```python
from build123d import *

# Parameters (mm, degrees)
SKETCH002_R      = 2.7
SKETCH002_R_2    = 1.4
EXTRUDE001_DEPTH = 7
EXTRUDE002_DEPTH = 23
EXTRUDE_DEPTH    = 1.6


with BuildPart() as obj1:
    # Sketch002 (on Face10 of Extrude) → Extrude001 (new body)
    with BuildSketch(Plane.XY.offset(-10.4)):
        with Locations((90.524621, -65.993824)):
            Circle(SKETCH002_R)
        with Locations((90.524621, -65.993824)):
            Circle(SKETCH002_R_2, mode=Mode.SUBTRACT)
        with Locations((90.502441, -92.471822)):
            Circle(SKETCH002_R)
        with Locations((90.502441, -92.471822)):
            Circle(SKETCH002_R_2, mode=Mode.SUBTRACT)
        with Locations((153.513474, -66.00515)):
            Circle(SKETCH002_R)
        with Locations((153.513474, -66.00515)):
            Circle(SKETCH002_R_2, mode=Mode.SUBTRACT)
        with Locations((153.502167, -92.48777)):
            Circle(SKETCH002_R)
        with Locations((153.502167, -92.48777)):
            Circle(SKETCH002_R_2, mode=Mode.SUBTRACT)
    extrude(amount=EXTRUDE001_DEPTH)


with BuildPart() as obj1_1:
    # Extrude001 placement: moved
    add(obj1.part.moved(Location((35, 0, 0))))


with BuildPart() as walls:
    # Sketch → Extrude002 (new body)
    with BuildSketch(Plane.XY):
        with BuildLine():
            Line((89.498192, -99.850084), (189.498192, -99.850084))
            ThreePointArc((189.498192, -99.850084), (194.165097, -97.916989), (196.098192, -93.250084))
            Line((196.098192, -93.250084), (196.098192, -65.250084))
            ThreePointArc((196.098192, -65.250084), (194.165097, -60.583179), (189.498192, -58.650084))
            Line((189.498192, -58.650084), (89.498192, -58.650084))
            ThreePointArc((89.498192, -58.650084), (84.831287, -60.583179), (82.898192, -65.250084))
            Line((82.898192, -65.250084), (82.898192, -93.250084))
            ThreePointArc((82.898192, -93.250084), (84.831287, -97.916989), (89.498192, -99.850084))
        make_face()
        with BuildLine():
            Line((89.498192, -60.250084), (189.498192, -60.250084))
            ThreePointArc((194.498192, -65.250084), (193.033726, -61.71455), (189.498192, -60.250084))
            Line((194.498192, -65.250084), (194.498192, -93.250084))
            ThreePointArc((189.498192, -98.250084), (193.033726, -96.785618), (194.498192, -93.250084))
            Line((189.498192, -98.250084), (89.498192, -98.250084))
            ThreePointArc((84.498192, -93.250084), (85.962658, -96.785618), (89.498192, -98.250084))
            Line((84.498192, -93.250084), (84.498192, -65.250084))
            ThreePointArc((89.498192, -60.250084), (85.962658, -61.71455), (84.498192, -65.250084))
        make_face(mode=Mode.SUBTRACT)
    extrude(amount=EXTRUDE002_DEPTH)


with BuildPart() as walls_1:
    # Extrude002 placement: moved
    add(walls.part.moved(Location((0, 0, -10.4))))


with BuildPart() as doos:
    # Sketch001 → Extrude (new body)
    with BuildSketch(Plane.XY):
        with BuildLine():
            Line((89.498192, -99.850084), (189.498192, -99.850084))
            ThreePointArc((189.498192, -99.850084), (194.165097, -97.916989), (196.098192, -93.250084))
            Line((196.098192, -93.250084), (196.098192, -65.250084))
            ThreePointArc((196.098192, -65.250084), (194.165097, -60.583179), (189.498192, -58.650084))
            Line((189.498192, -58.650084), (89.498192, -58.650084))
            ThreePointArc((89.498192, -58.650084), (84.831287, -60.583179), (82.898192, -65.250084))
            Line((82.898192, -65.250084), (82.898192, -93.250084))
            ThreePointArc((82.898192, -93.250084), (84.831287, -97.916989), (89.498192, -99.850084))
        make_face()
    extrude(amount=EXTRUDE_DEPTH)


with BuildPart() as doos_1:
    # Extrude placement: moved
    add(doos.part.moved(Location((0, 0, -12))))

    # Fusion: union obj1, Walls
    add(obj1_1.part)
    add(walls_1.part)


solid = doos_1.part
```
Source: CAD feature listing. Evaluate the final solid. Frame: model axes, mm. A direction names the side the tool comes from. Round coordinates to 2 decimals unless told otherwise and drop trailing zeros. Order: outer loops, then holes, each group sorted by start corner. A loop starts at its lowest first (then second) coordinate and runs counter-clockwise, first axis right, second up. Notation, with made-up numbers: (24.5, -10.5) -> (44.5, -10.5) arc R31 cw to (44.5, 18.5) -> close; hole circle Ø1 at (-6.5, -5.75). An arc over 180 degrees is marked (long way). Use CSV: the item, a comma, the result in double quotes.
(1) Pull-direction query (X, two-part tool) for faces 3 (the face through (125, -92, -10.4)), 4 (the face through (140, -58.65, 0)), 5 (the face through (84.78, -97.865, 0.128)); classes: +X half, -X half, draft (parallel to the pull), parting line (faces both ways), or undercut.
Report:
face 3,"undercut"
face 4,"draft"
face 5,"-X half"
(2) Ray query, L1, parallel to Y at x = 153, z = -6.75; L2, parallel to X at y = -66, z = 1.5; L3, parallel to Z at x = 160.5, y = -66. Return the intervals inside material, ascending.
Report:
L1,"-99.85 to -98.25, -60.25 to -58.65"
L2,"82.9 to 84.5, 194.5 to 196.1"
L3,"-12 to -10.4"
(3) Access query for faces 1 (the face through (82.898, -79, 0)), 2 (the face through (187.115, -65.944, -6.949)). Directions: +Z, -Z, +X, -X, +Y, -Y. A direction counts if a zero-diameter tool reaches every point of the face in a straight line with its end or side. Return the directions, or none.
Report:
face 1,"+Z, -Z, -X, +Y, -Y"
face 2,"+Z"
(4) Section D-D on x = 143. Return the cut outline in (y, z).
Report:
outline,"(-99.85, -12) -> (-58.65, -12) -> (-58.65, 12.6) -> (-60.25, 12.6) -> (-60.25, -10.4) -> (-98.25, -10.4) -> (-98.25, 12.6) -> (-99.85, 12.6) -> close"
(5) Section B-B on z = -5.75. Count the separate pieces of the cut face and the enclosed holes in it, and give its area (3 significant figures).
Report:
separate pieces,"5"
enclosed holes,"5"
area,"535 mm^2"
(6) Section C-C on y = -84. Return the cut outline in (x, z), and give its area (3 significant figures).
Report:
outline,"(82.9, -12) -> (196.1, -12) -> (196.1, 12.6) -> (194.5, 12.6) -> (194.5, -10.4) -> (84.5, -10.4) -> (84.5, 12.6) -> (82.9, 12.6) -> close"
area,"255 mm^2"
(7) Section A-A on z = 2.5. Return the cut outline in (x, y), and give its area (3 significant figures).
Report:
outline,"(82.9, -93.25) arc R6.6 ccw to (89.5, -99.85) -> (189.5, -99.85) arc R6.6 ccw to (196.1, -93.25) -> (196.1, -65.25) arc R6.6 ccw to (189.5, -58.65) -> (89.5, -58.65) arc R6.6 ccw to (82.9, -65.25) -> close; hole (84.5, -93.25) arc R5 ccw to (89.5, -98.25) -> (189.5, -98.25) arc R5 ccw to (194.5, -93.25) -> (194.5, -65.25) arc R5 ccw to (189.5, -60.25) -> (89.5, -60.25) arc R5 ccw to (84.5, -65.25) -> close"
area,"468 mm^2"
(8) First-contact query: pin 1 Ø2.5 at (x, y) = (189.5, -66) entering from +Z; pin 2 Ø8 at (x, y) = (157.5, -80) entering from +Z; pin 3 Ø4 at (y, z) = (-95.5, -0.5) entering from +X. Flat tips, straight axial feed; report the tip coordinate or a pass-through.
Report:
pin 1,"z = -3.4"
pin 2,"z = -10.4"
pin 3,"x = 196.09"
